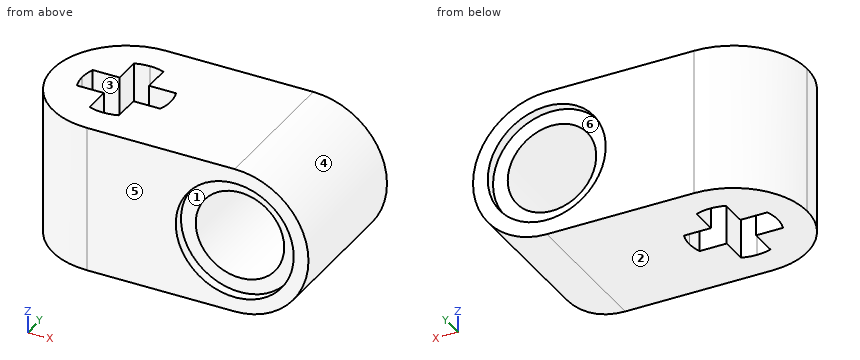
from build123d import *

# Parameters (mm, degrees)
SKETCH1_R           = 2.5
SKETCH1_R_2         = 2
SKETCH1_R_3         = 1.5
BOSS_EXTRUDE1_DEPTH = 5
SKETCH1_3_R         = 2
SKETCH1_3_R_2       = 1.5
CUT_EXTRUDE1_DEPTH  = 0.333333333
SKETCH2_R           = 2
SKETCH2_R_2         = 1.5
CUT_EXTRUDE2_DEPTH  = 0.333333333
CUT_EXTRUDE3_REACH  = 7
SKETCH3_W           = 1
SKETCH3_H           = 1


with BuildPart() as part:
    # Sketch1 → Boss-Extrude1 (new body)
    with BuildSketch(Plane(origin=(0, 0, 0), x_dir=(1, 0, 0), z_dir=(0, 1, 0))):
        with BuildLine():
            Line((-5, 2.5), (-5, -2.5))
            Line((-5, -2.5), (2.5, -2.5))
            ThreePointArc((2.5, -2.5), (0, 0), (2.5, 2.5))
            Line((2.5, 2.5), (-5, 2.5))
        make_face()
        with Locations((2.5, 0)):
            Circle(SKETCH1_R)
        with Locations((2.5, 0)):
            Circle(SKETCH1_R_2, mode=Mode.SUBTRACT)
        with Locations((2.5, 0)):
            Circle(SKETCH1_R_2)
        with Locations((2.5, 0)):
            Circle(SKETCH1_R_3, mode=Mode.SUBTRACT)
    extrude(amount=BOSS_EXTRUDE1_DEPTH)

    # Sketch1<3> → Cut-Extrude1 (cut)
    with BuildSketch(Plane(origin=(0, 0, 0), x_dir=(1, 0, 0), z_dir=(0, 1, 0))):
        with Locations((2.5, 0)):
            Circle(SKETCH1_3_R)
        with Locations((2.5, 0)):
            Circle(SKETCH1_3_R_2, mode=Mode.SUBTRACT)
    extrude(amount=CUT_EXTRUDE1_DEPTH, mode=Mode.SUBTRACT)

    # Sketch2 → Cut-Extrude2 (cut)
    with BuildSketch(Plane(origin=(0, 5, 0), x_dir=(1, 0, 0), z_dir=(0, 1, 0))):
        with Locations((2.5, 0)):
            Circle(SKETCH2_R)
        with Locations((2.5, 0)):
            Circle(SKETCH2_R_2, mode=Mode.SUBTRACT)
    extrude(amount=-CUT_EXTRUDE2_DEPTH, mode=Mode.SUBTRACT)

    # Sketch3 → Cut-Extrude3 (cut, up to next)
    with BuildSketch(Plane.XY.offset(2.5), mode=Mode.PRIVATE) as cut_extrude3_sk1:
        with BuildLine():
            Line((-2.5, 5), (-5, 5))
            Line((-5, 5), (-5, 2.5))
            ThreePointArc((-5, 2.5), (-4.267766953, 4.267766953), (-2.5, 5))
        make_face()
    cut_extrude3_tool1 = extrude(cut_extrude3_sk1.sketch, amount=-CUT_EXTRUDE3_REACH, mode=Mode.PRIVATE) & part.part
    add(cut_extrude3_tool1.solids().sort_by_distance((-4.44158, 4.44158, 2.5))[0], mode=Mode.SUBTRACT)
    # Sketch3 → Cut-Extrude3 (cut, up to next)
    with BuildSketch(Plane.XY.offset(2.5), mode=Mode.PRIVATE) as cut_extrude3_sk2:
        with BuildLine():
            ThreePointArc((-2.5, 0), (-4.267766953, 0.732233047), (-5, 2.5))
            Line((-5, 2.5), (-5, 0))
            Line((-5, 0), (-2.5, 0))
        make_face()
    cut_extrude3_tool2 = extrude(cut_extrude3_sk2.sketch, amount=-CUT_EXTRUDE3_REACH, mode=Mode.PRIVATE) & part.part
    add(cut_extrude3_tool2.solids().sort_by_distance((-4.44158, 0.55842, 2.5))[0], mode=Mode.SUBTRACT)
    # Sketch3 → Cut-Extrude3 (cut, up to next)
    with BuildSketch(Plane.XY.offset(2.5), mode=Mode.PRIVATE) as cut_extrude3_sk3:
        with BuildLine():
            Line((-3.914213562, 2), (-3, 2))
            Line((-3, 2), (-3, 3))
            Line((-3, 3), (-3.914213562, 3))
            ThreePointArc((-3.914213562, 3), (-3.978397839, 2.753652968), (-4, 2.5))
            ThreePointArc((-4, 2.5), (-3.978397839, 2.246347032), (-3.914213562, 2))
        make_face()
    cut_extrude3_tool3 = extrude(cut_extrude3_sk3.sketch, amount=-CUT_EXTRUDE3_REACH, mode=Mode.PRIVATE) & part.part
    add(cut_extrude3_tool3.solids().sort_by_distance((-3.486204, 2.5, 2.5))[0], mode=Mode.SUBTRACT)
    # Sketch3 → Cut-Extrude3 (cut, up to next)
    with BuildSketch(Plane.XY.offset(2.5), mode=Mode.PRIVATE) as cut_extrude3_sk4:
        with BuildLine():
            Line((-3, 3.914213562), (-3, 3))
            Line((-3, 3), (-2, 3))
            Line((-2, 3), (-2, 3.914213562))
            ThreePointArc((-2, 3.914213562), (-2.246347032, 3.978397839), (-2.5, 4))
            ThreePointArc((-2.5, 4), (-2.753652968, 3.978397839), (-3, 3.914213562))
        make_face()
    cut_extrude3_tool4 = extrude(cut_extrude3_sk4.sketch, amount=-CUT_EXTRUDE3_REACH, mode=Mode.PRIVATE) & part.part
    add(cut_extrude3_tool4.solids().sort_by_distance((-2.5, 3.486204, 2.5))[0], mode=Mode.SUBTRACT)
    # Sketch3 → Cut-Extrude3 (cut, up to next)
    with BuildSketch(Plane.XY.offset(2.5), mode=Mode.PRIVATE) as cut_extrude3_sk5:
        with Locations((-2.5, 2.5)):
            Rectangle(SKETCH3_W, SKETCH3_H)
    cut_extrude3_tool5 = extrude(cut_extrude3_sk5.sketch, amount=-CUT_EXTRUDE3_REACH, mode=Mode.PRIVATE) & part.part
    add(cut_extrude3_tool5.solids().sort_by_distance((-2.5, 2.5, 2.5))[0], mode=Mode.SUBTRACT)
    # Sketch3 → Cut-Extrude3 (cut, up to next)
    with BuildSketch(Plane.XY.offset(2.5), mode=Mode.PRIVATE) as cut_extrude3_sk6:
        with BuildLine():
            Line((-2, 3), (-2, 2))
            Line((-2, 2), (-1.085786438, 2))
            ThreePointArc((-1.085786438, 2), (-1.021602161, 2.246347032), (-1, 2.5))
            ThreePointArc((-1, 2.5), (-1.021602161, 2.753652968), (-1.085786438, 3))
            Line((-1.085786438, 3), (-2, 3))
        make_face()
    cut_extrude3_tool6 = extrude(cut_extrude3_sk6.sketch, amount=-CUT_EXTRUDE3_REACH, mode=Mode.PRIVATE) & part.part
    add(cut_extrude3_tool6.solids().sort_by_distance((-1.513796, 2.5, 2.5))[0], mode=Mode.SUBTRACT)
    # Sketch3 → Cut-Extrude3 (cut, up to next)
    with BuildSketch(Plane.XY.offset(2.5), mode=Mode.PRIVATE) as cut_extrude3_sk7:
        with BuildLine():
            ThreePointArc((-3, 1.085786438), (-2.753652968, 1.021602161), (-2.5, 1))
            ThreePointArc((-2.5, 1), (-2.246347032, 1.021602161), (-2, 1.085786438))
            Line((-2, 1.085786438), (-2, 2))
            Line((-2, 2), (-3, 2))
            Line((-3, 2), (-3, 1.085786438))
        make_face()
    cut_extrude3_tool7 = extrude(cut_extrude3_sk7.sketch, amount=-CUT_EXTRUDE3_REACH, mode=Mode.PRIVATE) & part.part
    add(cut_extrude3_tool7.solids().sort_by_distance((-2.5, 1.513796, 2.5))[0], mode=Mode.SUBTRACT)


solid = part.part
The listing builds one solid part. Answer for the finished solid, in the listing's coordinates (mm). Face numbers are marked on the shaded views. A direction names the side the tool comes from. Give positions to 0.01 mm unless a question says otherwise; leave off trailing zeros. Write each loop counter-clockwise with the first axis right and the second up, starting at its lowest first coordinate (ties: lowest second). Pieces come first, ordered by that corner, then holes.
Item 1: Section B-B, the plane y = 3.2 is taken. Write down the section's boundary in (x, z), plus the area to 3 significant figures.
Item 2: Find the intervals of material crossed by line 1 along X through (y, z) = (2.5, 0); line 2 along Z through (x, y) = (2.5, 3.7); line 3 along X through (y, z) = (2.95, 1.2), in increasing order.
Item 3: Flat-ended cylindrical pins translate along their axes: P1, Ø1, axis at x = -3.5, z = 0.5, coming from the +Y side; P2, Ø1, axis at x = -3.5, z = 1, coming from the -Y side; P3, Ø1.5, axis at y = 1.5, z = 0, coming from the -X side. Find the tip coordinate at first contact, or state that the pin passes through.
Item 4: Determine the mould class of the marked faces 4, 5 and 6 for opening direction X: released by +X, released by -X, zero draft, split by the parting line, or undercut.
Item 5: Section C-C, the plane x = -1.5 is taken. Write down the section's boundary in (y, z), plus the area to 3 significant figures.
Item 6: Section D-D, the plane z = -0.6 is taken. Write down the section's boundary in (x, y), plus the area to 3 significant figures.
Item 7: Section A-A, the plane z = 0 is taken. Write down the section's boundary in (x, y).
Item 8: Which of the six approach directions +Z, -Z, +X, -X, +Y, -Y give full straight-line access (tool end or side, diameter ignored) to the marked faces 1, 2 and 3?
Completed:
1. outline: (-4.9, -2.5) - (-3, -2.5) - (-3, 2.5) - (-4.9, 2.5) - close; (-2, -2.5) - (2.5, -2.5) arc R2.5 ccw to (2.5, 2.5) - (-2, 2.5) - close; hole circle Ø3 at (2.5, 0)
1. area: 34.7 mm2
2. line 1: x = -5 to -4, -1 to 1, 4 to 5
2. line 2: z = -2.5 to -1.5, 1.5 to 2.5
2. line 3: x = -4.96 to -3.93, -1.07 to 1.6, 3.4 to 4.69
3. P1: stops at y = 4.95
3. P2: stops at y = 0.05
3. P3: stops at x = -4.99
4. face 4: released by +X
4. face 5: zero draft
4. face 6: undercut
5. outline: (0, -2.5) - (2, -2.5) - (2, 2.5) - (0, 2.5) - close; (3, -2.5) - (5, -2.5) - (5, 2.5) - (3, 2.5) - close
5. area: 20.0 mm2
6. outline: (-2.5, 0) - (0.59, 0) - (0.59, 0.33) - (1.13, 0.33) - (1.13, 4.67) - (0.59, 4.67) - (0.59, 5) - (-2.5, 5) arc R2.5 ccw to start; (3.87, 0.33) - (4.41, 0.33) - (4.41, 0) - (4.93, 0) - (4.93, 5) - (4.41, 5) - (4.41, 4.67) - (3.87, 4.67) - close; hole (-3.91, 2) - (-3, 2) - (-3, 1.09) arc R1.5 ccw to (-2, 1.09) - (-2, 2) - (-1.09, 2) arc R1.5 ccw to (-1.09, 3) - (-2, 3) - (-2, 3.91) arc R1.5 ccw to (-3, 3.91) - (-3, 3) - (-3.91, 3) arc R1.5 ccw to start
6. area: 27.6 mm2
7. outline: (-2.5, 0) - (0.5, 0) - (0.5, 0.33) - (1, 0.33) - (1, 4.67) - (0.5, 4.67) - (0.5, 5) - (-2.5, 5) arc R2.5 ccw to start; (4, 0.33) - (4.5, 0.33) - (4.5, 0) - (5, 0) - (5, 5) - (4.5, 5) - (4.5, 4.67) - (4, 4.67) - close; hole (-3.91, 2) - (-3, 2) - (-3, 1.09) arc R1.5 ccw to (-2, 1.09) - (-2, 2) - (-1.09, 2) arc R1.5 ccw to (-1.09, 3) - (-2, 3) - (-2, 3.91) arc R1.5 ccw to (-3, 3.91) - (-3, 3) - (-3.91, 3) arc R1.5 ccw to start
8. face 1: -Y
8. face 2: -Z, +X, -X, +Y, -Y
8. face 3: +Z, -Z
